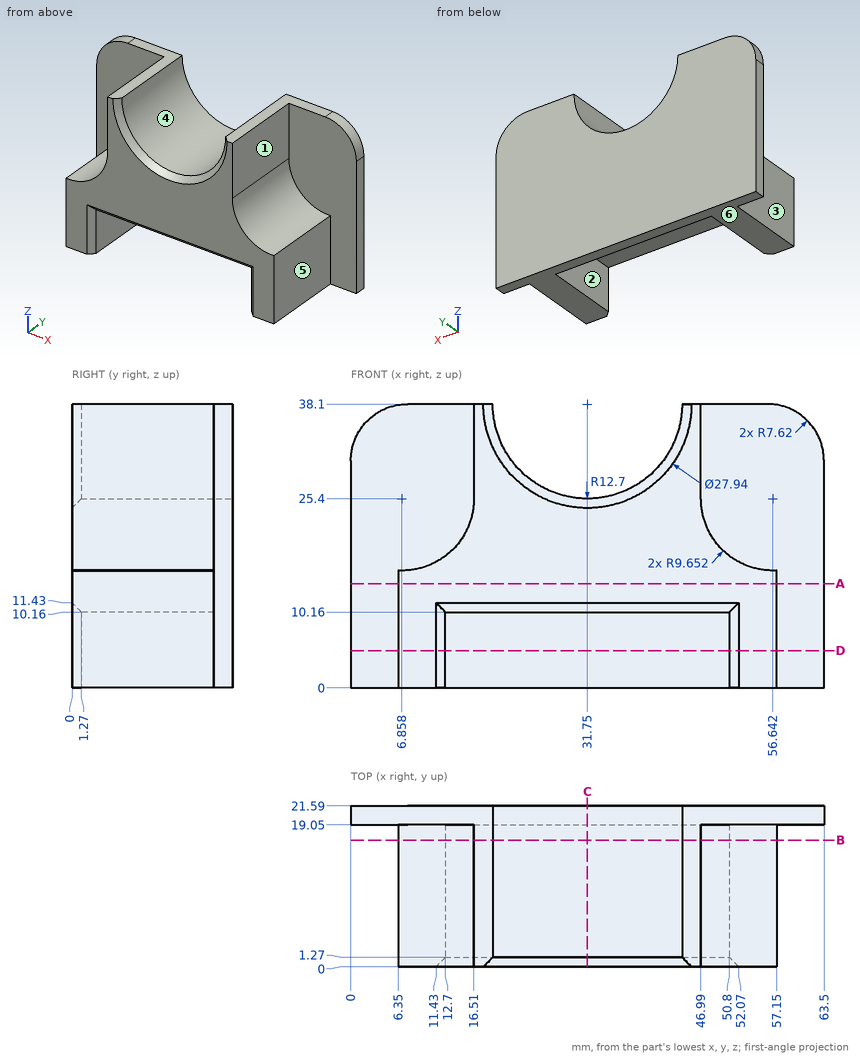
Could you check a few things on this drawing? It's one solid part, dimensions in mm from its lowest x, y, z. A direction names the side the tool comes from. Coordinates: 2 decimals unless noted, no trailing zeros. Order: outer loops, then holes, each group sorted by start corner. A loop starts at its lowest first (then second) coordinate and runs counter-clockwise, first axis right, second up. Notation, with made-up numbers: M 49.5,-13 L 69.5,-13 A11 cw 69.5,-1 Z; hole C 51.25,43.5 d3. An arc over 180 degrees is marked long. Use one line per item in the form item = value. Start each with the question number.
1. Suppose I cut it at C-C on x = 31.75. Write out the boundary of the cut face in (y, z).
2. We'd pull the mould along X, two halves only. Please class the marked faces 4, 5 and 6: +X half, -X half, draft (parallel to the pull), parting line (faces both ways), or undercut.
3. Please list where these lines run through material, in increasing order: line 1 (X direction, y = 1.5, z = 3); line 2 (Y direction, x = 31, z = 8); line 3 (X direction, y = 10.75, z = 13).
4. For pin 1 (12 mm diameter, centred on y = 8.5, z = 25, fed in from +X); pin 2 (8 mm diameter, centred on y = 11.5, z = 3.5, fed in from -X); pin 3 (5 mm diameter, centred on x = 26.5, z = 6, fed in from -Y), each with a flat end and sliding along its axis, tell me the tip position at first contact or that it passes through.
5. Suppose I cut it at A-A on z = 14. Write out the boundary of the cut face in (x, y), then the cut area to 3 significant figures.
6. Suppose I cut it at B-B on y = 17. Write out the boundary of the cut face in (x, z), then the cut area to 3 significant figures.
7. On a 3-axis mill with a long thin cutter (end or side, diameter ignored), from which of +Z, -Z, +X, -X, +Y, -Y can I reach the whole of each face in a straight line? I mean the marked faces 1, 2 and 3. Say none if no direction works.
8. Suppose I cut it at D-D on z = 5. Write out the boundary of the cut face in (x, y), then the cut area to 3 significant figures.
Geometry says:
q1.outline = M 0,11.43 L 1.27,10.16 L 19.05,10.16 L 19.05,0 L 21.59,0 L 21.59,25.4 L 1.27,25.4 L 0,24.13 Z
q2.face_4 = undercut
q2.face_5 = +X half
q2.face_6 = draft
q3.line_1 = 6.35 to 12.7, 50.8 to 57.15
q3.line_2 = 19.05 to 21.59
q3.line_3 = 6.35 to 57.15
q4.pin_1 = 49.42
q4.pin_2 = 6.35
q4.pin_3 = 19.05
q5.outline = M 0,19.05 L 6.35,19.05 L 6.35,0 L 57.15,0 L 57.15,19.05 L 63.5,19.05 L 63.5,21.59 L 0,21.59 Z
q5.area = 1,130 mm^2
q6.outline = M 6.35,0 L 12.7,0 L 12.7,10.16 L 50.8,10.16 L 50.8,0 L 57.15,0 L 57.15,15.76 A9.65 cw 46.99,25.4 L 46.99,38.1 L 44.45,38.1 A12.7 cw 19.05,38.1 L 16.51,38.1 L 16.51,25.4 A9.65 cw 6.35,15.76 Z
q6.area = 881 mm^2
q7.face_1 = +Z, +X, -Y
q7.face_2 = -Z, -Y
q7.face_3 = +Z, -Z, -X, -Y
q8.outline = M 0,19.05 L 6.35,19.05 L 6.35,0 L 11.43,0 L 12.7,1.27 L 12.7,19.05 L 50.8,19.05 L 50.8,1.27 L 52.07,0 L 57.15,0 L 57.15,19.05 L 63.5,19.05 L 63.5,21.59 L 0,21.59 Z
q8.area = 402 mm^2
